Part model, mm, in its own coordinate system. A direction names the side the tool comes from. Round coordinates to 2 decimals unless told otherwise and drop trailing zeros. Order: outer loops, then holes, each group sorted by start corner. A loop starts at its lowest first (then second) coordinate and runs counter-clockwise, first axis right, second up. Notation, with made-up numbers: (21.25, 50.25) -> (54.25, 50.25) arc R21 cw to (54.25, 69.25) -> close; hole circle Ø5 at (-17.5, 46). An arc over 180 degrees is marked (long way). Use CSV: the item, a comma, the result in double quotes.
```python
from build123d import *

# Parameters (mm, degrees)
SKETCH1_R               = 4.7
BOSS_EXTRUDE1_DEPTH     = 11.866666667
SKETCH2_OUTSIDE_W       = 14.964
SKETCH2_OUTSIDE_H       = 14.964
SKETCH2_OUTSIDE_R       = 1.85
CUT_EXTRUDE1_DEPTH      = 3.5
BOSS_EXTRUDE2_START     = -8.366666667
BOSS_EXTRUDE2_DEPTH     = 8.366666667
FILLET1_R               = 0.5
FILLET2_R               = 0.5
SKETCH4_R               = 2.4
BOSS_EXTRUDE3_DEPTH     = 8.5
FILLET3_R               = 1
CHAMFER1_SIZE           = 0.5
CUT_EXTRUDE2_DEPTH      = 22.816361088
CUT_EXTRUDE2_DEPTH_BACK = 22.816361088
SKETCH5_R               = 1.275


with BuildPart() as part:
    # Sketch1 → Boss-Extrude1 (new body)
    with BuildSketch(Plane.XY):
        Circle(SKETCH1_R)
    extrude(amount=BOSS_EXTRUDE1_DEPTH)

    # Sketch2 outside → Cut-Extrude1 (cut)
    with BuildSketch(Plane(origin=(0, 0, 0), x_dir=(-1, 0, 0), z_dir=(0, 0, -1))):
        Rectangle(SKETCH2_OUTSIDE_W, SKETCH2_OUTSIDE_H)
        Circle(SKETCH2_OUTSIDE_R, mode=Mode.SUBTRACT)
    extrude(amount=-CUT_EXTRUDE1_DEPTH, mode=Mode.SUBTRACT)

    # Sketch3 → Boss-Extrude2 (add)
    with BuildSketch(Plane.XY.offset(11.866666667).offset(BOSS_EXTRUDE2_START)):
        with BuildLine():
            Line((-1, 6.16948134), (-1, 4.592385001))
            ThreePointArc((-1, 4.592385001), (0, 4.7), (1, 4.592385001))
            Line((1, 4.592385001), (1, 6.16948134))
            ThreePointArc((1, 6.16948134), (0, 6.25), (-1, 6.16948134))
        make_face()
        with BuildLine():
            ThreePointArc((1, -4.592385001), (0, -4.7), (-1, -4.592385001))
            Line((-1, -4.592385001), (-1, -6.16948134))
            ThreePointArc((-1, -6.16948134), (0, -6.25), (1, -6.16948134))
            Line((1, -6.16948134), (1, -4.592385001))
        make_face()
    extrude(amount=BOSS_EXTRUDE2_DEPTH)

    # Fillet1
    fillet1_edges = [part.edges().sort_by_distance(p)[0] for p in [
        (-1, 6.16948134, 7.683333333),
        (-1, 4.592385001, 7.683333333),
        (1, 4.592385001, 7.683333333),
        (1, 6.16948134, 7.683333333),
        (1, -6.16948134, 7.683333333),
        (1, -4.592385001, 7.683333333),
        (-1, -4.592385001, 7.683333333),
        (-1, -6.16948134, 7.683333333),
    ]]
    fillet(fillet1_edges, radius=FILLET1_R)

    # Fillet2
    fillet2_edges = [part.edges().sort_by_distance(p)[0] for p in [
        (1.85, 0, 3.5),
    ]]
    fillet(fillet2_edges, radius=FILLET2_R)

    # Sketch4 → Boss-Extrude3 (add)
    with BuildSketch(Plane.XY.offset(11.866666667)):
        Circle(SKETCH4_R)
    extrude(amount=BOSS_EXTRUDE3_DEPTH)

    # Fillet3
    fillet3_edges = [part.edges().sort_by_distance(p)[0] for p in [
        (-2.4, 0, 11.866666667),
    ]]
    fillet(fillet3_edges, radius=FILLET3_R)

    # Chamfer1
    chamfer1_edges = [part.edges().sort_by_distance(p)[0] for p in [
        (1.85, 0, 0),
        (-2.4, 0, 20.366666667),
    ]]
    chamfer(chamfer1_edges, length=CHAMFER1_SIZE)

    # Sketch5 → Cut-Extrude2 (cut, two sides: drawn at the far end of the back side and taken through both)
    with BuildSketch(Plane(origin=(0, 0, 0), x_dir=(1, 0, 0), z_dir=(0, 1, 0)).offset(-CUT_EXTRUDE2_DEPTH_BACK)):
        with Locations(Location((0, -16.841666667, 0), (0, 0, 270))):
            Circle(SKETCH5_R)
    extrude(amount=CUT_EXTRUDE2_DEPTH + CUT_EXTRUDE2_DEPTH_BACK, mode=Mode.SUBTRACT)


solid = part.part
```
(1) Pull direction X, two halves, no side cores. Call faces 4 (the face through (0.06, -0.03, 15.57)), 5 (the face through (-1.77, 1.62, 16.32)), 6 (the face through (4.7, -0.1, 7.6)), 7 (the face through (0, 0, 0)): released by +X, released by -X, zero draft, split by the parting line, or undercut.
Reply:
face 4,"undercut"
face 5,"split by the parting line"
face 6,"released by +X"
face 7,"zero draft"
(2) Which spindle directions (+Z, -Z, +X, -X, +Y, -Y) get a long thin tool onto all of the face, cutting with end or side? Do faces 1 (the face through (0.401, -1.806, 1.732)), 2 (the face through (-4.7, 0.1, 7.6)), 3 (the face through (-2, 3, 11.867)). Say none if no direction does.
Reply:
face 1,"-Z"
face 2,"+Z, -Z, -X"
face 3,"+Z"
(3) Cut at D-D, the plane z = 14. Give the cut face in (x, y).
Reply:
outline,"circle Ø4.8 at (0, 0)"
(4) Cut at A-A, the plane x = 0. Give the cut face in (y, z).
Reply:
outline,"(-6.25, 3.5) -> (-2.35, 3.5) arc R0.5 cw to (-1.85, 3) -> (-1.85, 0.5) -> (-1.35, 0) -> (1.35, 0) -> (1.85, 0.5) -> (1.85, 3) arc R0.5 cw to (2.35, 3.5) -> (6.25, 3.5) -> (6.25, 11.87) -> (3.4, 11.87) arc R1 cw to (2.4, 12.87) -> (2.4, 15.57) -> (-2.4, 15.57) -> (-2.4, 12.87) arc R1 cw to (-3.4, 11.87) -> (-6.25, 11.87) -> close; (-2.4, 18.12) -> (2.4, 18.12) -> (2.4, 19.87) -> (1.9, 20.37) -> (-1.9, 20.37) -> (-2.4, 19.87) -> close"
(5) Cut at C-C, the plane y = 0. Give the cut face in (x, z) (3 decimals).
Reply:
outline,"(-4.7, 3.5) -> (-2.35, 3.5) arc R0.5 cw to (-1.85, 3) -> (-1.85, 0.5) -> (-1.35, 0) -> (1.35, 0) -> (1.85, 0.5) -> (1.85, 3) arc R0.5 cw to (2.35, 3.5) -> (4.7, 3.5) -> (4.7, 11.867) -> (3.4, 11.867) arc R1 cw to (2.4, 12.867) -> (2.4, 19.867) -> (1.9, 20.367) -> (-1.9, 20.367) -> (-2.4, 19.867) -> (-2.4, 12.867) arc R1 cw to (-3.4, 11.867) -> (-4.7, 11.867) -> close; hole circle Ø2.55 at (0, 16.842)"
(6) Drop flat-ended pins along their axis: P1, Ø1, axis at y = 3, z = 13.5, coming from the -X side; P2, Ø1.5, axis at x = -3.5, z = 6, coming from the +Y side; P3, Ø5, axis at y = 4.5, z = 5, coming from the -X side; P4, Ø3, axis at x = 0, z = 16.84, coming from the +Y side. Give the stop position or say it passes through.
Reply:
P1,"through"
P2,"y = 3.81"
P3,"x = -4.25"
P4,"y = 2.4"
(7) Probe probe 1 along Z at (x, y) = (0, 0.15); probe 2 along Y at (x, z) = (0.5, 7); probe 3 along X at (y, z) = (3.25, 10.25). List the from-to ranges inside material, lowest first. Write a range as [from, to].
Reply:
probe 1,"[0, 15.57], [18.12, 20.37]"
probe 2,"[-6.23, 6.23]"
probe 3,"[-3.4, 3.4]"
(8) Cut at B-B, the plane z = 11.5. Give the cut face in (x, y), then the cut area to 3 significant figures.
Reply:
outline,"(-1.36, -4.5) arc R0.5 cw to (-1, -4.98) -> (-1, -5.73) arc R0.5 ccw to (-0.54, -6.23) arc R6.25 ccw to (0.54, -6.23) arc R0.5 ccw to (1, -5.73) -> (1, -4.98) arc R0.5 cw to (1.36, -4.5) arc R4.7 ccw to (1.36, 4.5) arc R0.5 cw to (1, 4.98) -> (1, 5.73) arc R0.5 ccw to (0.54, 6.23) arc R6.25 ccw to (-0.54, 6.23) arc R0.5 ccw to (-1, 5.73) -> (-1, 4.98) arc R0.5 cw to (-1.36, 4.5) arc R4.7 ccw to start"
area,"75.6 mm2"
